Part print with two shaded views. Sizes in mm from the minimum x, y, z corner. A direction names the side the tool comes from. Coordinates: 2 decimals unless noted, no trailing zeros. Write each loop counter-clockwise with the first axis right and the second up, starting at its lowest first coordinate (ties: lowest second). Pieces come first, ordered by that corner, then holes.
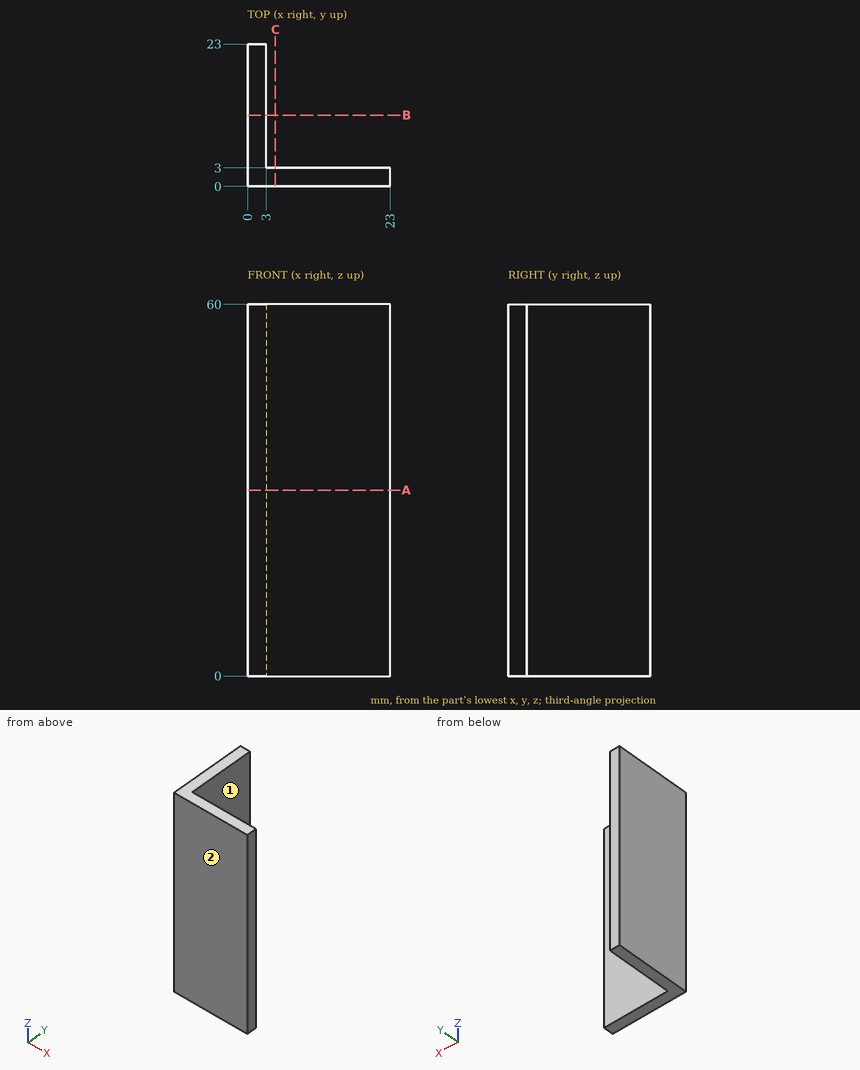
(1) Slice it at B-B, the plane y = 11.5. List the corners of the cut face in (x, z), and give its area (3 significant figures).
(2) Probe L1, parallel to Y at x = 16, z = 6. List the from-to ranges inside material, lowest first.
(3) Flat gauge pins, fed straight in: P1, Ø1, axis at y = 7, z = 17, coming from the -X side; P2, Ø3, axis at x = 20.5, z = 52, coming from the +Y side. Where does each tip first touch, or does it go through?
(4) 3-axis set-ups, long thin cutter, end or side, ignore diameter. For the marked faces 1 and 2: which of +Z, -Z, +X, -X, +Y, -Y reach the whole face in a straight line?
(5) Slice it at A-A, the plane z = 30. List the corners of the cut face in (x, y), and give its area (3 significant figures).
Results:
1. outline: (0, 0) - (3, 0) - (3, 60) - (0, 60) - close
1. area: 180 mm2
2. L1: y = 0 to 3
3. P1: stops at x = 0
3. P2: stops at y = 3
4. face 1: +Z, -Z, +X, +Y
4. face 2: +Z, -Z, +X, -X, -Y
5. outline: (0, 0) - (23, 0) - (23, 3) - (3, 3) - (3, 23) - (0, 23) - close
5. area: 129 mm2
